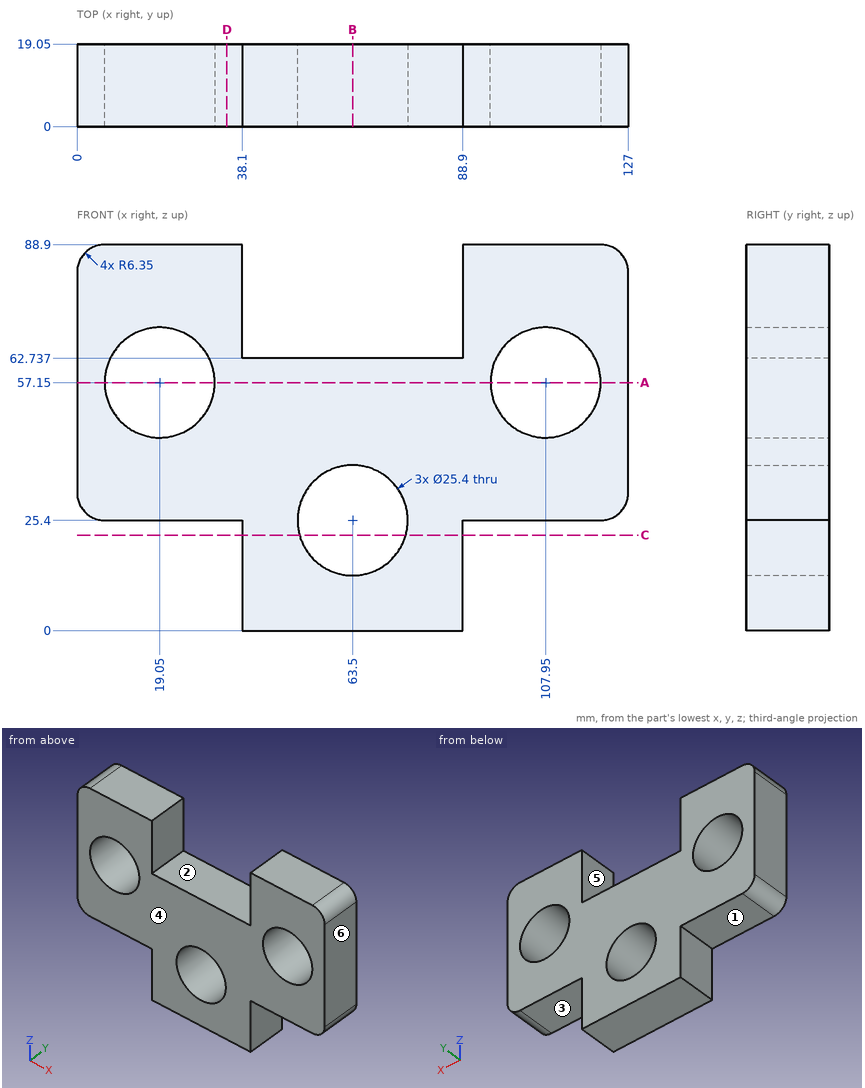
Geometry check sheet. Reference: drawing and pictorial views, mm from the part's lowest x, y, z. A direction names the side the tool comes from. Give positions to 0.01 mm unless a question says otherwise; leave off trailing zeros. Order: outer loops, then holes, each group sorted by start corner. A loop starts at its lowest first (then second) coordinate and runs counter-clockwise, first axis right, second up.
1. Access from +Z, -Z, +X, -X, +Y, -Y to the whole of each face (thin tool, end or side, straight path). Record for the marked faces 1, 2 and 3.
2. Gauge pin test, flat ends, axial feed: pin 1 Ø3 at (x, y) = (97, 7) entering from -Z; pin 2 Ø5.5 at (y, z) = (6.5, 10) entering from +X; pin 3 Ø2 at (x, y) = (68, 9) entering from +Z. Record the tip position at first contact, or that the pin passes through.
3. Section check A-A, the plane z = 57.15. Enter the section's corners in (x, y).
4. Section check C-C, the plane z = 22. Enter the section's corners in (x, y), and give its area (3 significant figures).
5. Section check B-B, the plane x = 63.5. Enter the section's corners in (y, z).
6. Release check for a two-part mould opening along X. For the marked faces 4, 5 and 6 record: pulls with the +X half, pulls with the -X half, needs draft (parallel to the pull), parting line crosses it, or undercut.
7. Thickness scan on L1, parallel to Z at x = 107.95, y = 7.5; L2, parallel to Z at x = 63.5, y = 4; L3, parallel to X at y = 5.75, z = 78.5. Record the ranges inside material, lowest first.
8. Section check D-D, the plane x = 34.5. Enter the section's corners in (y, z), and give its area (3 significant figures).
Values follow:
1. face 1: -Z, -X, +Y, -Y
1. face 2: +Z, +Y, -Y
1. face 3: -Z, +X, +Y, -Y
2. pin 1: stops at z = 25.4
2. pin 2: stops at x = 88.9
2. pin 3: stops at z = 62.74
3. outline: (0, 0) - (6.35, 0) - (6.35, 19.05) - (0, 19.05) - close; (31.75, 0) - (95.25, 0) - (95.25, 19.05) - (31.75, 19.05) - close; (120.65, 0) - (127, 0) - (127, 19.05) - (120.65, 19.05) - close
4. outline: (38.1, 0) - (51.26, 0) - (51.26, 19.05) - (38.1, 19.05) - close; (75.74, 0) - (88.9, 0) - (88.9, 19.05) - (75.74, 19.05) - close
4. area: 502 mm2
5. outline: (0, 0) - (19.05, 0) - (19.05, 12.7) - (0, 12.7) - close; (0, 38.1) - (19.05, 38.1) - (19.05, 62.74) - (0, 62.74) - close
6. face 4: needs draft
6. face 5: undercut
6. face 6: pulls with the +X half
7. L1: z = 25.4 to 44.45, 69.85 to 88.9
7. L2: z = 0 to 12.7, 38.1 to 62.74
7. L3: x = 0 to 38.1, 88.9 to 127
8. outline: (0, 25.4) - (19.05, 25.4) - (19.05, 88.9) - (0, 88.9) - close
8. area: 1,210 mm2
